The figure shows three views and two pictorial views of one solid part (mm, origin at its lowest corner). Answer the questions. A direction names the side the tool comes from. Round coordinates to 2 decimals unless told otherwise and drop trailing zeros. Order: outer loops, then holes, each group sorted by start corner. A loop starts at its lowest first (then second) coordinate and runs counter-clockwise, first axis right, second up.
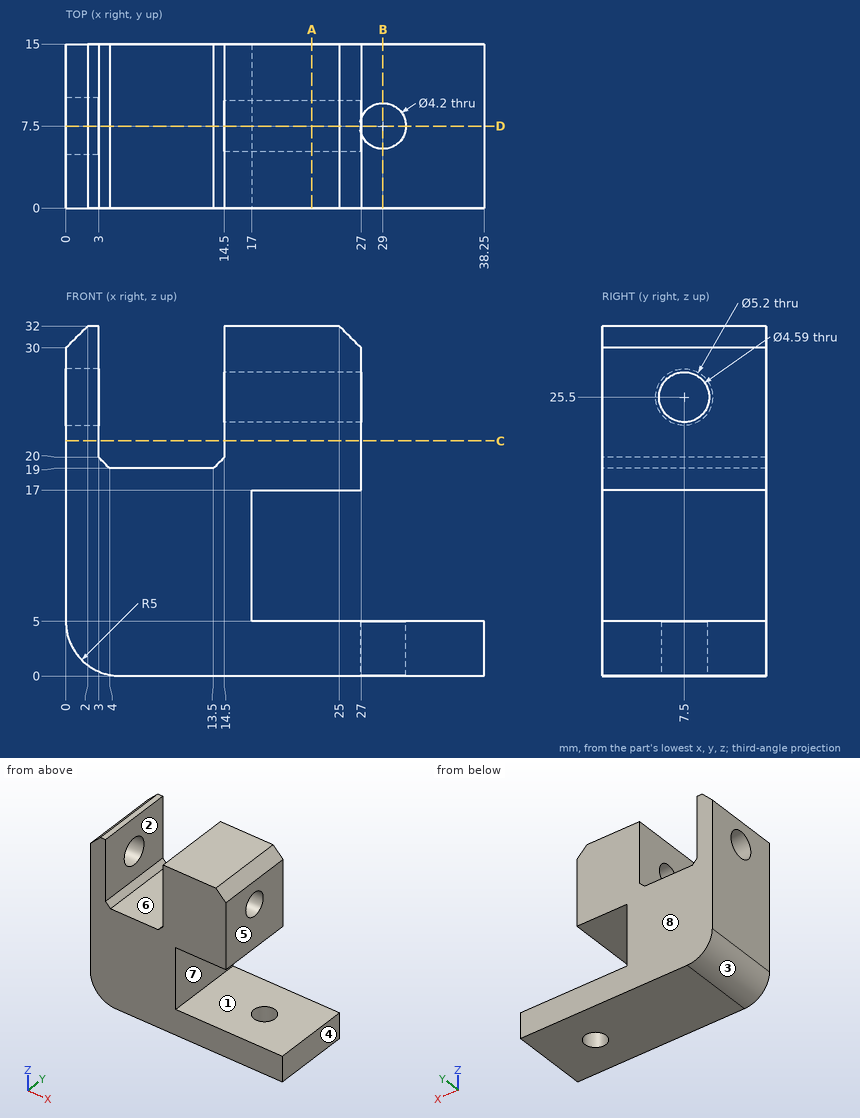
Item 1: Find section A-A (x = 22.5). Write down the section's boundary in (y, z) (3 decimals).
Item 2: A tool of negligible diameter and unlimited length cuts with its end or side. For the marked faces 4, 5, 6, 7 and 8, from which of +Z, -Z, +X, -X, +Y, -Y can it reach the whole face along a straight path? Write none if from no direction.
Item 3: For a pull along Z with two mould halves and no side action, classify the marked faces 1, 2 and 3 as released by +Z, released by -Z, zero draft, split by the parting line, or undercut.
Item 4: Given pin 1 (5 mm diameter, centred on x = 9, y = 10, fed in from +Z); pin 2 (5.5 mm diameter, centred on x = 29, y = 7.5, fed in from +Z); pin 3 (6 mm diameter, centred on y = 6.5, z = 9, fed in from +X), each flat-ended and moving along its own axis, determine where each tip first touches the part or whether it passes through.
Item 5: Find the intervals of material crossed by line 1 along Z through (x, y) = (17.75, 7.5) (3 decimals); line 2 along X through (y, z) = (13.75, 28); line 3 along X through (y, z) = (1, 14.5), in increasing order.
Item 6: Find section D-D (y = 7.5). State how many separate pieces and enclosed holes the cut face has, plus the area to 3 significant figures.
Item 7: Find section B-B (x = 29). Write down the section's boundary in (y, z), plus the area to 3 significant figures.
Item 8: Find section C-C (z = 21.5). Write down the section's boundary in (x, y), plus the area to 4 significant figures.
Model answer:
1. outline: (0, 0) - (15, 0) - (15, 5) - (0, 5) - close; (0, 17) - (15, 17) - (15, 32) - (0, 32) - close; hole circle Ø4.59 at (7.5, 25.5)
2. face 4: +Z, -Z, +X, +Y, -Y
2. face 5: +Z, +X, +Y, -Y
2. face 6: +Z, +Y, -Y
2. face 7: +X, +Y, -Y
2. face 8: +Z, -Z, +X, -X, +Y
3. face 1: undercut
3. face 2: zero draft
3. face 3: released by -Z
4. pin 1: stops at z = 19
4. pin 2: stops at z = 30.75
4. pin 3: stops at x = 17
5. line 1: z = 0 to 5, 17 to 23.205, 27.795 to 32
5. line 2: x = 0 to 3, 14.5 to 27
5. line 3: x = 0 to 17
6. separate pieces: 4
6. enclosed holes: 0
6. area: 548 mm2
7. outline: (0, 0) - (5.4, 0) - (5.4, 5) - (0, 5) - close; (9.6, 0) - (15, 0) - (15, 5) - (9.6, 5) - close
7. area: 54.0 mm2
8. outline: (0, 0) - (3, 0) - (3, 15) - (0, 15) - close; (14.5, 0) - (27, 0) - (27, 15) - (14.5, 15) - close
8. area: 232.5 mm2
